Could you check a few things on this model? Use its own coordinates, in mm. Round coordinates to 2 decimals unless told otherwise and drop trailing zeros. Loops run counter-clockwise (first coordinate to the right, second up) from the corner with the lowest first, then second, coordinate; pieces in that order, holes last. Notation, with made-up numbers: (52.25, 78.5) - (103.25, 78.5) arc R23 ccw to (103.25, 92.5) - close; hole circle Ø10 at (7.5, 11.25). An arc over 180 degrees is marked (long way). Put each result on its own line as item: value. Start each with the question number.
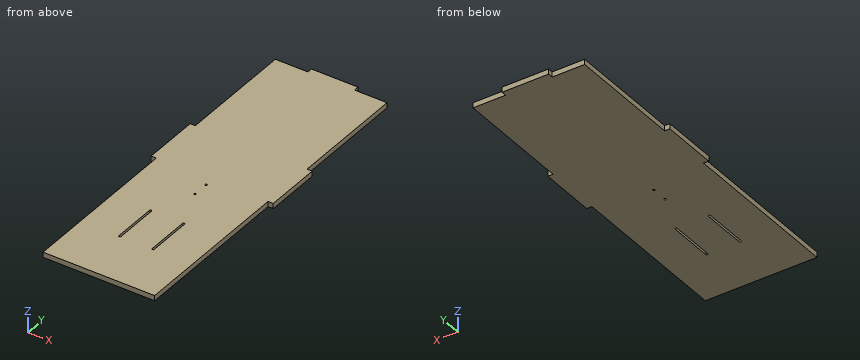
Autodesk Inventor part; units mm, degrees
ref_plane "YZ Plane" through (0, 0, 0) normal (1, 0, 0) x (0, 1, 0)
ref_plane "XZ Plane" through (0, 0, 0) normal (0, 1, 0) x (-1, 0, 0)
ref_plane "XY Plane" through (0, 0, 0) normal (0, 0, 1) x (1, 0, 0)
sketch "Sketch1" plane through (0, 0, 0) normal (0, 0, 1) x (1, 0, 0)
  line L0 (-75, 93.8197) -> (75, 93.8197)
  line L1 (75, 93.8197) -> (75, -336.1803)
  line L2 (75, -336.1803) -> (-75, -336.1803)
  line L3 (-75, -336.1803) -> (-75, 93.8197)
  point P0 (0, 0)
  dimension "d0" = 150
  dimension "d1" = 430
extrude "Extrusion1" add sketch "Sketch1" along normal blind 6.35
sketch "Sketch2" plane through (0, 0, 6.35) normal (0, 0, 1) x (1, 0, 0)
  line L0 (75, 93.8197) -> (-75, 93.8197)
  line L1 (-75, 93.8197) -> (-68.65, 93.8197)
  line L2 (-68.65, 93.8197) -> (-68.65, -56.1803)
  line L3 (-68.65, -56.1803) -> (-75, -56.1803)
  line L4 (-75, -56.1803) -> (-75, 93.8197)
  line L5 (-75, 93.8197) -> (-75, -336.1803)
  line L6 (-75, -126.1803) -> (-68.65, -126.1803)
  line L7 (-68.65, -126.1803) -> (-68.65, -236.1803)
  line L8 (-68.65, -236.1803) -> (-75, -236.1803)
  line L9 (-75, -236.1803) -> (-75, -126.1803)
  line L10 (-75, 93.8197) -> (-75, -336.1803)
  line L11 (-75, -336.1803) -> (-68.65, -336.1803)
  line L12 (-68.65, -336.1803) -> (-68.65, -186.1803)
  line L13 (-68.65, -186.1803) -> (-75, -186.1803)
  line L14 (-75, -186.1803) -> (-75, -336.1803)
  line L15 (75, -336.1803) -> (75, 93.8197)
  line L16 (75, 93.8197) -> (68.65, 93.8197)
  line L17 (68.65, 93.8197) -> (68.65, -56.1803)
  line L18 (68.65, -56.1803) -> (75, -56.1803)
  line L19 (75, -56.1803) -> (75, 93.8197)
  line L20 (75, -126.1803) -> (68.65, -126.1803)
  line L21 (68.65, -126.1803) -> (68.65, -236.1803)
  line L22 (68.65, -236.1803) -> (75, -236.1803)
  line L23 (75, -236.1803) -> (75, -126.1803)
  line L24 (-75, -336.1803) -> (75, -336.1803)
  line L25 (75, -336.1803) -> (68.65, -336.1803)
  line L26 (68.65, -336.1803) -> (68.65, -186.1803)
  line L27 (68.65, -186.1803) -> (75, -186.1803)
  line L28 (75, -186.1803) -> (75, -336.1803)
  line L29 (-68.65, 93.8197) -> (-28.65, 93.8197)
  line L30 (-28.65, 93.8197) -> (-28.65, 87.4697)
  line L31 (-28.65, 87.4697) -> (-68.65, 87.4697)
  line L32 (-68.65, 87.4697) -> (-68.65, 93.8197)
  line L33 (68.65, 93.8197) -> (28.65, 93.8197)
  line L34 (28.65, 93.8197) -> (28.65, 87.4697)
  line L35 (28.65, 87.4697) -> (68.65, 87.4697)
  line L36 (68.65, 87.4697) -> (68.65, 93.8197)
  line L37 (-68.65, -336.1803) -> (68.9785, -336.1803)
  line L38 (68.9785, -336.1803) -> (68.9785, -329.8303)
  line L39 (-68.65, -329.8303) -> (-68.65, -336.1803)
  line L40 (68.65, -329.8303) -> (68.65, -336.1803)
  line L41 (-75, -336.1803) -> (75, -336.1803)
  line L42 (75, -336.1803) -> (75, -329.8303)
  line L43 (75, -329.8303) -> (-75, -329.8303)
  line L44 (-75, -329.8303) -> (-75, -336.1803)
  point P0 (0, 0)
  point P1 (-75, -186.1803)
  point P2 (75, -186.1803)
  point P3 (-75, -236.1803)
  point P4 (75, -236.1803)
  point P5 (75, -126.1803)
  point P6 (75, -56.1803)
  dimension "d4" = 150
  dimension "d5" = 110
  dimension "d6" = 150
  dimension "d7" = 70
  dimension "d8" = 6.35
  dimension "d9" = 6.35
  dimension "d12" = 6.35
  dimension "d13" = 6.35
  dimension "d14" = 40
  dimension "d15" = 40
  dimension "d32" = 150
  dimension "d33" = 150
  dimension "d34" = 110
  dimension "d35" = 70
  dimension "d36" = 6.35
extrude "Extrusion2" cut sketch "Sketch2" against normal through all contours L15 L18 L17 L0 | L17 L35 L34 L0 | L15 L27 L21 L20 | L30 L31 L2 L0 | L15 L22 L21 L27 | L2 L3 L4 L0 | L15 L43 L26 L22 | L15 L24 L38 L43 | L38 L24 L26 L43 | L26 L24 L12 L43 | L6 L7 L13 L5 | L43 L5 L8 L12 | L12 L11 L5 L43 | L13 L7 L8 L5
sketch "Sketch4" plane through (0, 0, 6.35) normal (0, 0, 1) x (1, 0, 0)
  circle A0 centre (0, -157.1803) radius 1.25
  line L0 (-68.65, -336.1803) -> (68.65, -336.1803)
  line L1 (28.65, 93.8197) -> (-28.65, 93.8197)
  circle A1 centre (0, -137.1803) radius 1.25
  line L2 (0, -207.1803) -> (20.41, -207.1803)
  circle A2 centre (20.41, -207.1803) radius 1.25
  line L3 (0, -207.1803) -> (-20.41, -207.1803)
  circle A3 centre (-20.41, -207.1803) radius 1.25
  line L4 (0, -137.1803) -> (-75, -137.1803)
  line L5 (-75, -56.1803) -> (-75, -126.1803)
  line L6 (-75, -137.1803) -> (-75, -126.1803)
  line L7 (0, -157.1803) -> (0, -137.1803)
  line L8 (0, -207.1803) -> (0, -157.1803)
  circle A4 centre (-20.41, -262.1803) radius 1.25
  circle A5 centre (20.41, -262.1803) radius 1.25
  line L9 (-21.66, -262.1803) -> (-21.66, -207.1803)
  line L10 (-19.16, -262.1803) -> (-19.16, -207.1803)
  line L11 (19.16, -262.1803) -> (19.16, -207.1803)
  line L12 (21.66, -207.1803) -> (21.66, -262.1803)
  line L13 (21.66, -262.1803) -> (19.16, -262.1803)
  line L14 (-75, -56.1803) -> (-75, -126.1803)
  point P0 (0, 0)
  point P1 (-28.65, -336.1803)
  point P2 (28.65, -336.1803)
  point P3 (-75, -236.1803)
  point P4 (-75, -306.1803)
  dimension "d18" = 2.5
  dimension "d22" = 251
  dimension "d23" = 20
  dimension "d25" = 20.41
  dimension "d26" = 75
  dimension "d27" = 50
  dimension "d28" = 55
  dimension "d30" = 55
  dimension "d31" = 55
extrude "Extrusion3" cut sketch "Sketch4" against normal through all
equation "\"d9\" = d8"
equation "\"d13\" = d8"
equation "\"d15\" = d14"
equation "\"d32\" = d4"
equation "\"d33\" = d6"
equation "\"d34\" = d5"
equation "\"d35\" = d7"
equation "\"d30\" = d28"
properties part number "2201_Housing Bottom_V1" material "Wood (Birch)"
Item 1: Will these pins go through, and if not, where does the flat tip stop? P1, Ø1.9, axis at y = -226, z = 1.5, coming from the -X side; P2, Ø1.5, axis at x = -1.5, y = 34.5, coming from the -Z side; P3, Ø2, axis at y = 34, z = 5.5, coming from the +X side; P4, Ø3, axis at x = 73, z = 2, coming from the +Y side.
Item 2: Suppose I cut it at B-B, the plane z = 4.5. List the corners of the cut face in (x, y) for me.
Item 3: Suppose I cut it at A-A, the plane y = -217. List the corners of the cut face in (x, z) for me.
Item 4: Suppose I cut it at C-C, the plane y = -33.5. List the corners of the cut face in (x, z) for me, then the cut area to 3 significant figures.
Item 5: I need wall thicknesses on line 1 (Y direction, x = 0, z = 2.25); line 2 (X direction, y = -247.5, z = 5.5); line 3 (X direction, y = 61, z = 1). Which ranges of each line are inside material? Lowest first, please. Write a range as from..to.
Numbers:
1. P1: x = -68.65
1. P2: z = 0
1. P3: x = 68.65
1. P4: y = -56.18
2. outline: (-75, -126.18) - (-68.65, -126.18) - (-68.65, -329.83) - (68.65, -329.83) - (68.65, -126.18) - (75, -126.18) - (75, -56.18) - (68.65, -56.18) - (68.65, 87.47) - (28.65, 87.47) - (28.65, 93.82) - (-28.65, 93.82) - (-28.65, 87.47) - (-68.65, 87.47) - (-68.65, -56.18) - (-75, -56.18) - close; hole (-21.66, -262.18) arc R1.25 ccw to (-19.16, -262.18) - (-19.16, -207.18) arc R1.25 ccw to (-21.66, -207.18) - close; hole circle Ø2.5 at (0, -157.18); hole circle Ø2.5 at (0, -137.18); hole (19.16, -262.18) arc R1.25 ccw to (21.66, -262.18) - (21.66, -207.18) arc R1.25 ccw to (19.16, -207.18) - close
3. outline: (-68.65, 0) - (-21.66, 0) - (-21.66, 6.35) - (-68.65, 6.35) - close; (-19.16, 0) - (19.16, 0) - (19.16, 6.35) - (-19.16, 6.35) - close; (21.66, 0) - (68.65, 0) - (68.65, 6.35) - (21.66, 6.35) - close
4. outline: (-68.65, 0) - (68.65, 0) - (68.65, 6.35) - (-68.65, 6.35) - close
4. area: 872 mm^2
5. line 1: -329.83..-158.43, -155.93..-138.43, -135.93..93.82
5. line 2: -68.65..-21.66, -19.16..19.16, 21.66..68.65
5. line 3: -68.65..68.65
